Read the model definition and answer for the solid it produces. Units are mm, in the model's axes. Face numbers are marked on the shaded views. A direction names the side the tool comes from. Round coordinates to 2 decimals unless told otherwise and drop trailing zeros. Order: outer loops, then holes, each group sorted by start corner. A loop starts at its lowest first (then second) coordinate and runs counter-clockwise, first axis right, second up.
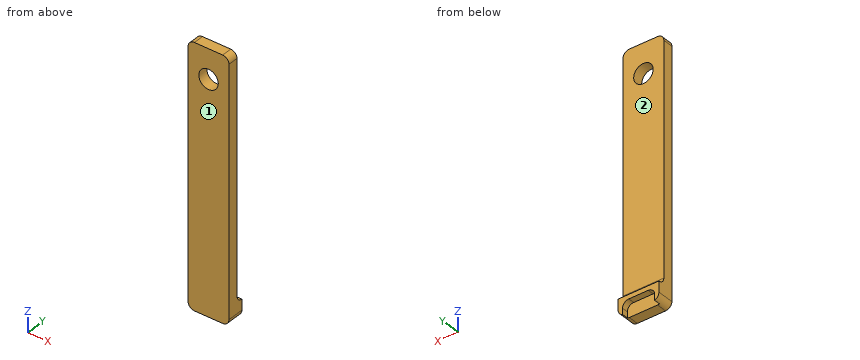
from build123d import *

# Parameters (mm, degrees)
SKETCH1_W           = 6.5
SKETCH1_H           = 41.15
SKETCH1_R           = 1.55
BOSS_EXTRUDE1_DEPTH = 1.65
BOSS_EXTRUDE2_DEPTH = 1
FILLET1_R           = 1


with BuildPart() as part:
    # Sketch1 → Boss-Extrude1 (new body)
    with BuildSketch(Plane(origin=(0, 0, 0), x_dir=(1, 0, 0), z_dir=(0, 1, 0))):
        with Locations((3.25, 20.575)):
            Rectangle(SKETCH1_W, SKETCH1_H)
        with Locations(Location((3.25, 4.7, 0), (0, 0, 270))):
            Circle(SKETCH1_R, mode=Mode.SUBTRACT)
    extrude(amount=BOSS_EXTRUDE1_DEPTH)

    # Sketch2 → Boss-Extrude2 (add)
    with BuildSketch(Plane(origin=(0, 1.65, 0), x_dir=(1, 0, 0), z_dir=(0, 1, 0))):
        Polygon((0, 41.15), (0.7, 41.15), (0.7, 39.15), (5.8, 39.15), (5.8, 41.15), (6.5, 41.15), (6.5, 39.15), (6.5, 38.45), (0, 38.45), (0, 39.15), align=None)
    extrude(amount=BOSS_EXTRUDE2_DEPTH)

    # Fillet1
    fillet1_edges = [part.edges().sort_by_distance(p)[0] for p in [
        (6.5, 1.325, -41.15),
        (0, 1.325, -41.15),
        (6.5, 0.825, 0),
        (0, 0.825, 0),
        (3.25, 1.65, -38.45),
        (0.7, 2.15, -39.15),
        (5.8, 2.15, -39.15),
    ]]
    fillet(fillet1_edges, radius=FILLET1_R - 0.0001)  # a hair under: the kernel refuses the full size


solid = part.part
Q1. A cutting plane is placed at D-D, the plane y = 2.3. Give the vertices of the cut face in (x, z).
Outcome:
outline: (0, -40.15) arc R1 ccw to (0.7, -41.1) - (0.7, -40.15) arc R1 cw to (1.7, -39.15) - (4.8, -39.15) arc R1 cw to (5.8, -40.15) - (5.8, -41.1) arc R1 ccw to (6.5, -40.15) - (6.5, -38.39) - (0, -38.39) - close
Q2. Straight lines are drawn through the part: probe 1 along X at (y, z) = (0.55, -4.7); probe 2 along Y at (x, z) = (2.5, -12); probe 3 along Z at (x, y) = (2.25, 0.3). For each, find the intervals that lie inside material, in ascending order.
Outcome:
probe 1: x = 0 to 1.7, 4.8 to 6.5
probe 2: y = 0 to 1.65
probe 3: z = -41.15 to -5.88, -3.52 to 0
Q3. A cutting plane is placed at B-B, the plane y = 0.8. Give the vertices of the cut face in (x, z).
Outcome:
outline: (0, -40.15) arc R1 ccw to (1, -41.15) - (5.5, -41.15) arc R1 ccw to (6.5, -40.15) - (6.5, -1) arc R1 ccw to (5.5, 0) - (1, 0) arc R1 ccw to (0, -1) - close; hole circle Ø3.1 at (3.25, -4.7)
Q4. For the marked faces 1 and 2, determine the directions among +Z, -Z, +X, -X, +Y, -Y from which every point of the face is accessible in a straight line to the end or side of a thin tool.
Outcome:
face 1: +Z, -Z, +X, -X, -Y
face 2: +Z, +X, -X, +Y
Q5. A cutting plane is placed at C-C, the plane z = -4.7. Give the vertices of the cut face in (x, y).
Outcome:
outline: (0, 0) - (1.7, 0) - (1.7, 1.65) - (0, 1.65) - close; (4.8, 0) - (6.5, 0) - (6.5, 1.65) - (4.8, 1.65) - close
Q6. Flat-ended cylindrical pins translate along their axes: pin 1 (1.6 mm diameter, centred on x = 4, z = -40.5, fed in from +Y); pin 2 (0.5 mm diameter, centred on y = 2, z = -40.5, fed in from -X) (3 decimals); pin 3 (2.5 mm diameter, centred on x = 3.25, z = -4.7, fed in from -Y); pin 4 (3 mm diameter, centred on x = 4, z = -30.5, fed in from -Y). Find the tip coordinate at first contact, or state that the pin passes through.
Outcome:
pin 1: stops at y = 1.65
pin 2: stops at x = 0.005
pin 3: passes through
pin 4: stops at y = 0
